```python
from build123d import *

# Parameters (mm, degrees)
F1_DEPTH = 9.906
F2_R     = 12.300458
F3_DEPTH = 101.6
F5_DEPTH = 6.096


with BuildPart() as f1:
    # F0 (on Top) → F1 (new body)
    with BuildSketch(Plane.XY):
        Polygon((-87.349732, 14.484886), (-157.059993, 7.486077), (-171.945385, -60.975071), (-111.434803, -96.287578), (-59.151814, -49.65076), align=None)
    extrude(amount=F1_DEPTH)

    # F2 (on face) → F3 (join)
    with BuildSketch(Plane(origin=(0, 0, 0), x_dir=(1, 0, 0), z_dir=(0, 0, -1))):
        with Locations((-119.881563, 38.058758)):
            Circle(F2_R)
    extrude(amount=F3_DEPTH)

    # F4 (on face) → F5 (join)
    with BuildSketch(Plane(origin=(0, 0, -101.6), x_dir=(1, 0, 0), z_dir=(0, 0, -1))):
        Polygon((-139.301867, 11.329003), (-100.461259, 11.329003), (-88.458851, 48.268616), (-119.881563, 71.098552), (-151.304275, 48.268616), align=None)
    extrude(amount=F5_DEPTH)


solid = f1.part
```
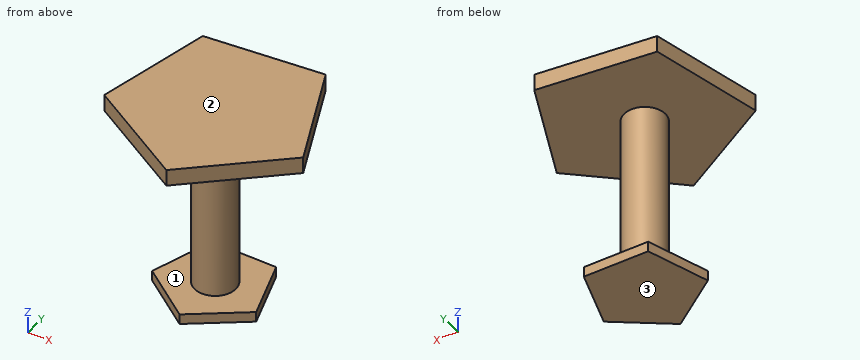
Could you check a few things on this model? Use its own coordinates, in mm. Face numbers are marked on the shaded views. Round coordinates to 2 decimals unless told otherwise and drop trailing zeros. Order: outer loops, then holes, each group sorted by start corner. A loop starts at its lowest first (then second) coordinate and runs counter-clockwise, first axis right, second up. Notation, with made-up numbers: (-23, -19) -> (4, -19) arc R32 cw to (4, 19) -> close; hole circle Ø6 at (45, -24.5). An arc over 180 degrees is marked (long way). One line per question, with ' | ' between items.
Q1. If we section it at B-B on x = -96.5: Write out the boundary of the cut face in (y, z).
Computed values:
outline: (-82.97, 0) -> (13.57, 0) -> (13.57, 9.91) -> (-82.97, 9.91) -> close; (-54.11, -107.7) -> (-23.52, -107.7) -> (-23.52, -101.6) -> (-54.11, -101.6) -> close
Q2. If we section it at C-C on y = -31: Write out the boundary of the cut face in (x, z).
Computed values:
outline: (-165.43, 0) -> (-129.96, 0) -> (-129.96, -101.6) -> (-145.69, -101.6) -> (-145.69, -107.7) -> (-94.07, -107.7) -> (-94.07, -101.6) -> (-109.81, -101.6) -> (-109.81, 0) -> (-67.35, 0) -> (-67.35, 9.91) -> (-165.43, 9.91) -> close
Q3. We'd pull the mould along Z, two halves only. Please class the marked faces 1, 2 and 3: released by +Z, released by -Z, zero draft, split by the parting line, or undercut.
Computed values:
face 1: undercut | face 2: released by +Z | face 3: released by -Z
Q4. If we section it at A-A on y = -17: Write out the boundary of the cut face in (x, z), plus the area to 3 significant figures.
Computed values:
outline: (-162.38, 0) -> (-73.51, 0) -> (-73.51, 9.91) -> (-162.38, 9.91) -> close; (-141.14, -107.7) -> (-98.62, -107.7) -> (-98.62, -101.6) -> (-141.14, -101.6) -> close | area: 1,140 mm²
Q5. If we section it at D-D on x = -115: Write out the boundary of the cut face in (y, z).
Computed values:
outline: (-94.21, 0) -> (-49.35, 0) -> (-49.35, -101.6) -> (-67.55, -101.6) -> (-67.55, -107.7) -> (-11.33, -107.7) -> (-11.33, -101.6) -> (-26.77, -101.6) -> (-26.77, 0) -> (11.71, 0) -> (11.71, 9.91) -> (-94.21, 9.91) -> close
Q6. I'm going to push flat-ended pins straight in: pin 1 (8 mm diameter, centred on x = -113.5, z = -23, fed in from +Y); pin 2 (1.8 mm diameter, centred on x = -114.5, z = -106, fed in from +Y); pin 3 (10 mm diameter, centred on y = -47, z = -69, fed in from +X). Where does each tip first touch, or does it pass through?
Computed values:
pin 1: y = -25.99 | pin 2: y = -11.33 | pin 3: x = -108.23
Q7. If I drill on line 1 (Z direction, x = -118, y = -21.5); line 2 (Z direction, x = -89, y = -15.5); line 3 (X direction, y = -35.5, z = -63.5), over which ranges is the centre line in solid material (lowest first)? Write a range as from..to.
Computed values:
line 1: -107.7..-101.6, 0..9.91 | line 2: 0..9.91 | line 3: -131.91..-107.85
